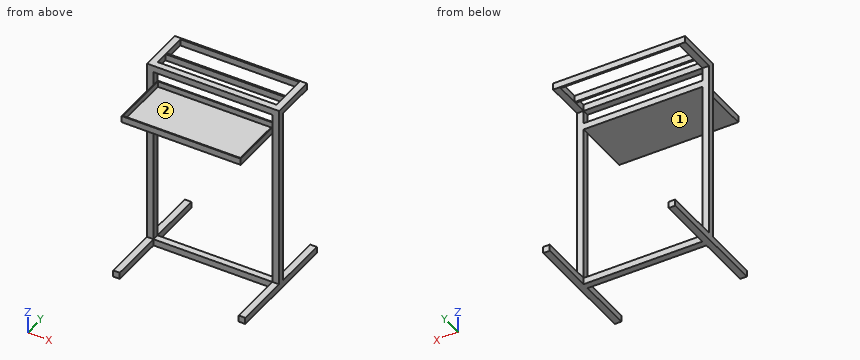
from build123d import *

# Parameters (mm, degrees)
F0_W     = 457.2
F0_H     = 25.4
F1_DEPTH = 25.4
F2_W     = 25.4
F2_H     = 25.4
F3_DEPTH = 711.2
F4_W     = 457.2
F4_H     = 6.35
F5_DEPTH = 25.4
F6_W     = 228.6
F6_H     = 25.4
F6_W_2   = 25.4
F7_DEPTH = 457.2
F8_W     = 450.85
F8_H     = 222.25
F9_DEPTH = 22.225


with BuildPart() as f1:
    # F0 (on Top) → F1 (new body)
    with BuildSketch(Plane.XY):
        Polygon((0, 457.2), (0, 0), (25.4, 0), (25.4, 215.9), (25.4, 241.3), (25.4, 457.2), align=None)
        with Locations((254, 228.6)):
            Rectangle(F0_W, F0_H)
        Polygon((482.6, 241.3), (482.6, 215.9), (482.6, 0), (508, 0), (508, 457.2), (482.6, 457.2), align=None)
    extrude(amount=F1_DEPTH)

    # F2 (on face) → F3 (join)
    with BuildSketch(Plane.XY.offset(25.4)):
        with Locations((12.7, 228.6)):
            Rectangle(F2_W, F2_H)
        with Locations((495.3, 228.6)):
            Rectangle(F2_W, F2_H)
    extrude(amount=F3_DEPTH)

    # F4 (on face) → F5 (join)
    with BuildSketch(Plane.XY.offset(736.6)):
        Polygon((0, 393.7), (0, 241.3), (25.4, 241.3), (25.4, 292.1), (25.4, 298.45), (25.4, 342.9), (25.4, 349.25), (25.4, 387.35), (25.4, 393.7), align=None)
        with Locations((254, 295.275)):
            Rectangle(F4_W, F4_H)
        with Locations((254, 390.525)):
            Rectangle(F4_W, F4_H)
        Polygon((482.6, 298.45), (482.6, 292.1), (482.6, 241.3), (508, 241.3), (508, 393.7), (482.6, 393.7), (482.6, 387.35), (482.6, 349.25), (482.6, 342.9), align=None)
    extrude(amount=-F5_DEPTH)

    # F6 (on face) → F7 (join, through all)
    with BuildSketch(Plane.YZ.offset(25.4)):
        with Locations((127, 647.7)):
            Rectangle(F6_W, F6_H)
        with Locations((228.6, 723.9)):
            Rectangle(F6_W_2, F6_H)
    extrude(amount=F7_DEPTH)

    # F8 (on face) → F9 (cut)
    with BuildSketch(Plane.XY.offset(660.4)):
        with Locations((254, 127)):
            Rectangle(F8_W, F8_H)
    extrude(amount=-F9_DEPTH, mode=Mode.SUBTRACT)


solid = f1.part
Model file for the job. Use its own axes, mm. Face numbers are marked on the shaded views. Give positions to 0.01 mm unless a question says otherwise; leave off trailing zeros. Order: outer loops, then holes, each group sorted by start corner. A loop starts at its lowest first (then second) coordinate and runs counter-clockwise, first axis right, second up. Notation, with made-up numbers: M 6.5,-10.5 L 18.5,-10.5 A11 cw 18.5,-2.5 Z; hole C 21.5,13.25 d10. An arc over 180 degrees is marked long. Put each result on its own line as item: value. Start each with the question number.
(1) Band-saw the part on C-C on z = 410.5. Give the cut face in (x, y), then the cut area to 3 significant figures.
(2) Band-saw the part on A-A on x = 319. Give the cut face in (y, z) (3 decimals), then the cut area to 3 significant figures.
(3) Band-saw the part on B-B on y = 125.5. Give the cut face in (x, z) (3 decimals), then the cut area to 3 significant figures.
(4) Drill centre lines: L1, parallel to X at y = 81, z = 642.5 (3 decimals); L2, parallel to Y at x = 23, z = 73; L3, parallel to Z at x = 337, y = 46 (3 decimals). Where is each one in solid material? Low to high. Write a range as [from, to].
(5) Pin check, flat tips, straight feed: pin 1 Ø11 at (x, z) = (355, 646) entering from +Y; pin 2 Ø10 at (x, z) = (184.5, 641.5) entering from -Y; pin 3 Ø7.5 at (x, z) = (260.5, 729) entering from +Y. Stop position of each tip, or through.
(6) Band-saw the part on D-D on y = 358. Give the cut face in (x, z), then the cut area to 3 significant figures.
(7) Pull direction Y, two halves, no side cores. Call the marked faces 1 and 2: released by +Y, released by -Y, zero draft, split by the parting line, or undercut.
Results below:
1. outline: M 0,215.9 L 25.4,215.9 L 25.4,241.3 L 0,241.3 Z; M 482.6,215.9 L 508,215.9 L 508,241.3 L 482.6,241.3 Z
1. area: 1,290 mm2
2. outline: M 12.7,635 L 241.3,635 L 241.3,660.4 L 238.125,660.4 L 238.125,638.175 L 15.875,638.175 L 15.875,660.4 L 12.7,660.4 Z; M 215.9,0 L 241.3,0 L 241.3,25.4 L 215.9,25.4 Z; M 215.9,711.2 L 241.3,711.2 L 241.3,736.6 L 215.9,736.6 Z; M 292.1,711.2 L 298.45,711.2 L 298.45,736.6 L 292.1,736.6 Z; M 387.35,711.2 L 393.7,711.2 L 393.7,736.6 L 387.35,736.6 Z
2. area: 2,480 mm2
3. outline: M 0,0 L 25.4,0 L 25.4,25.4 L 0,25.4 Z; M 25.4,635 L 482.6,635 L 482.6,660.4 L 479.425,660.4 L 479.425,638.175 L 28.575,638.175 L 28.575,660.4 L 25.4,660.4 Z; M 482.6,0 L 508,0 L 508,25.4 L 482.6,25.4 Z
3. area: 2,880 mm2
4. L1: x = [25.4, 28.575], [479.425, 482.6]
4. L2: y = [215.9, 241.3]
4. L3: z = [635, 638.175]
5. pin 1: stops at y = 241.3
5. pin 2: stops at y = 12.7
5. pin 3: stops at y = 393.7
6. outline: M 0,0 L 25.4,0 L 25.4,25.4 L 0,25.4 Z; M 0,711.2 L 25.4,711.2 L 25.4,736.6 L 0,736.6 Z; M 482.6,0 L 508,0 L 508,25.4 L 482.6,25.4 Z; M 482.6,711.2 L 508,711.2 L 508,736.6 L 482.6,736.6 Z
6. area: 2,580 mm2
7. face 1: zero draft
7. face 2: undercut
